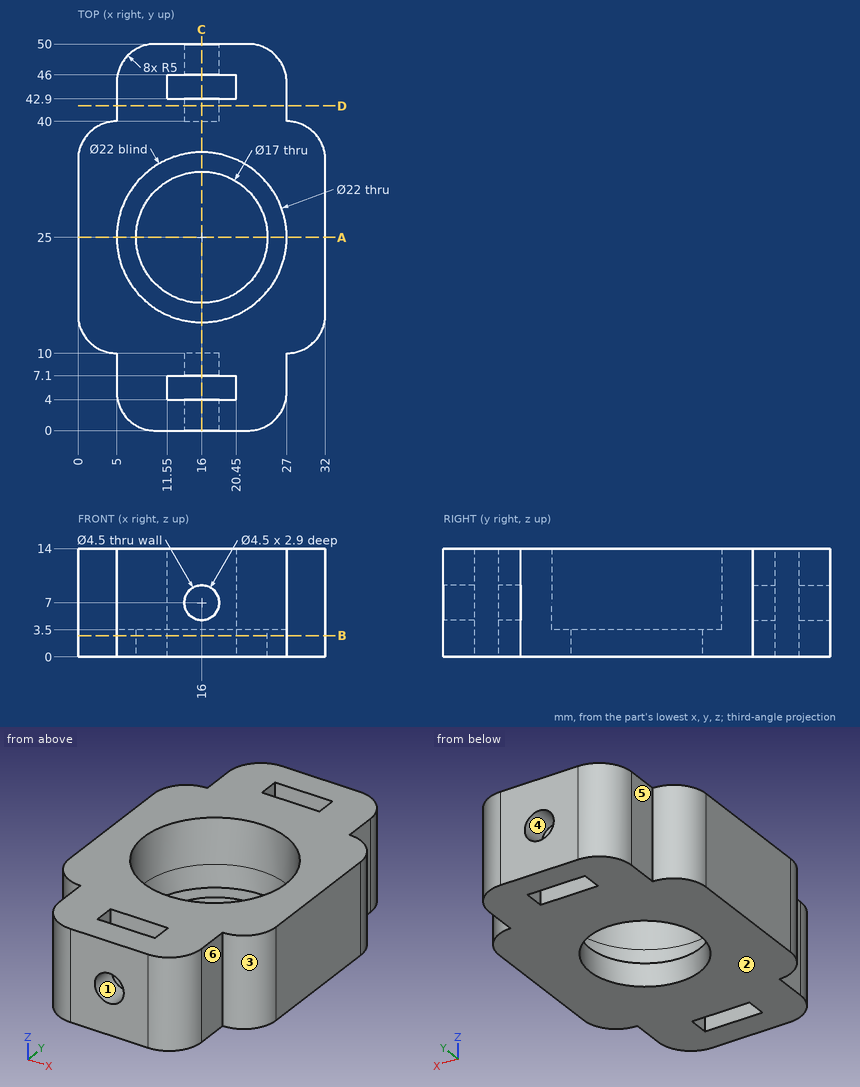
Input: dimensioned drawing with shaded views. Units: mm. Origin: part minimum x, y, z. A direction names the side the tool comes from. Give positions to 0.01 mm unless a question says otherwise; leave off trailing zeros. Write each loop counter-clockwise with the first axis right and the second up, starting at its lowest first coordinate (ties: lowest second). Pieces come first, ordered by that corner, then holes.
Q1. First-contact query: P1, Ø6, axis at x = 7.5, z = 11.5, coming from the +Y side; P2, Ø1.6, axis at y = 5, z = 4, coming from the +X side; P3, Ø3.5, axis at y = 5, z = 5.5, coming from the -X side; P4, Ø2, axis at x = 25.5, z = 1.5, coming from the +Y side. Flat tips, straight axial feed; report the tip coordinate or a pass-through.
Q2. Section A-A, the plane y = 25. Output: boundary loops of the cut face in (x, z), plus the area to 4 significant figures.
Q3. Pull-direction query (X, two-part tool) for the marked faces 1, 2 and 3; classes: pulls with the +X half, pulls with the -X half, needs draft (parallel to the pull), parting line crosses it, or undercut.
Q4. Section D-D, the plane y = 42. Output: boundary loops of the cut face in (x, z), plus the area to 3 significant figures.
Q5. Section C-C, the plane x = 16. State how many separate pieces and enclosed holes the cut face has, plus the area to 3 significant figures.
Q6. Section B-B, the plane z = 2.75. Output: boundary loops of the cut face in (x, y).
Q7. Material intervals for probe 1 along X at (y, z) = (24.5, 4); probe 2 along Y at (x, z) = (16, 6.2); probe 3 along Y at (x, z) = (12, 10.75), sorted ascending.
Q8. Set-up query: the marked faces 4, 5 and 6. Return all of +Z, -Z, +X, -X, +Y, -Y with unobstructed straight access to the full face (end or side cutting, diameter ignored); none if empty.
Filled in:
1. P1: stops at y = 50
1. P2: stops at x = 27
1. P3: stops at x = 5
1. P4: stops at y = 49.33
2. outline: (0, 0) - (7.5, 0) - (7.5, 3.5) - (5, 3.5) - (5, 14) - (0, 14) - close; (24.5, 0) - (32, 0) - (32, 14) - (27, 14) - (27, 3.5) - (24.5, 3.5) - close
2. area: 157.5 mm2
3. face 1: undercut
3. face 2: needs draft
3. face 3: pulls with the +X half
4. outline: (5, 0) - (27, 0) - (27, 14) - (5, 14) - close; hole circle Ø4.5 at (16, 7)
4. area: 292 mm2
5. separate pieces: 6
5. enclosed holes: 0
5. area: 261 mm2
6. outline: (0, 15) arc R5 ccw to (5, 10) - (5, 5) arc R5 ccw to (10, 0) - (22, 0) arc R5 ccw to (27, 5) - (27, 10) arc R5 ccw to (32, 15) - (32, 35) arc R5 ccw to (27, 40) - (27, 45) arc R5 ccw to (22, 50) - (10, 50) arc R5 ccw to (5, 45) - (5, 40) arc R5 ccw to (0, 35) - close; hole circle Ø17 at (16, 25); hole (11.55, 4) - (20.45, 4) - (20.45, 7.1) - (11.55, 7.1) - close; hole (11.55, 42.9) - (20.45, 42.9) - (20.45, 46) - (11.55, 46) - close
7. probe 1: x = 0 to 5.01, 26.99 to 32
7. probe 2: y = 10 to 14, 36 to 40
7. probe 3: y = 0 to 4, 7.1 to 14.75, 35.25 to 42.9, 46 to 50
8. face 4: +Y
8. face 5: +Z, -Z, -X, +Y
8. face 6: +Z, -Z, +X, -Y
